The model under review builds one solid part; all positions refer to its coordinate system, in mm. Face numbers are marked on the shaded views. Give positions to 0.01 mm unless a question says otherwise; leave off trailing zeros. Order: outer loops, then holes, each group sorted by start corner. A loop starts at its lowest first (then second) coordinate and runs counter-clockwise, first axis right, second up. Notation, with made-up numbers: (6.25, 33.25) -> (42.25, 33.25) arc R25 ccw to (42.25, 53.25) -> close; hole circle Ø9 at (80, -19). An arc over 180 degrees is marked (long way). Use one line per item in the form item = value.
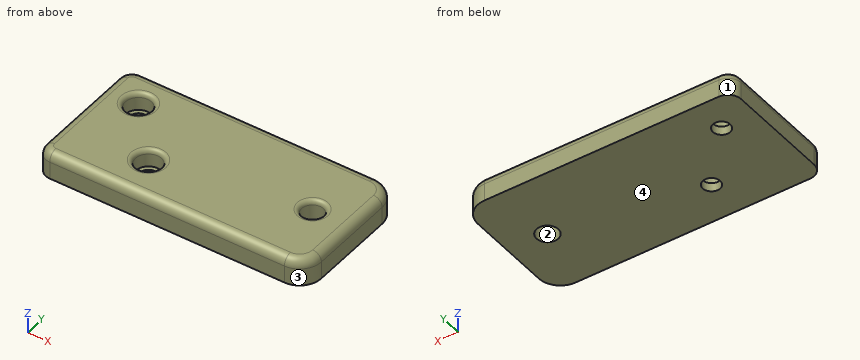
Autodesk Fusion 360 part; units mm, degrees
sketch "Sketch1" plane through (0, 0, 0) normal (0, 0, 1) x (1, 0, 0)
  circle A0 centre (0, 0) radius 2
  circle A1 centre (11.2624, -12.7341) radius 2
  circle A2 centre (11.2624, -12.7341) radius 3
  circle A3 centre (0, 0) radius 3
  line L0 (-8, 8) -> (54, 8)
  line L1 (54, 8) -> (54, -21.9327)
  line L2 (54, -21.9327) -> (-8, -21.9327)
  line L3 (-8, -21.9327) -> (-8, 8)
  circle A4 centre (45, -7) radius 2.5
  dimension "d1" = 4
  dimension "d2" = 4
  dimension "d3" = 6
  dimension "d4" = 6
  dimension "d5" = 17
  dimension "d6" = 5
extrude "Extrude1" add sketch "Sketch1" against normal blind 6 contours A2 | A3 | L0 L1 L2 L3
extrude "Extrude2" cut sketch "Sketch1" against normal blind 4 contours A2 | A3
fillet "Fillet1" radius 5 2 edges at (54, -21.9327, -3) (54, 8, -3)
fillet "Fillet2" radius 3 2 edges at (-8, -21.9327, -3) (-8, 8, -3)
fillet "Fillet3" radius 2 8 edges at (-8, -6.9663, 0) (-7.1213, 7.1213, 0) (22, 8, 0) (52.5355, 6.5355, 0) (54, -6.9663, 0) (52.5355, -20.4682, 0) (22, -21.9327, 0) (-7.1213, -21.054, 0)
fillet "Fillet4" radius 1 3 edges at (42.6692, -6.096, 0) (8.4654, -11.6493, 0) (-2.797, 1.0848, 0)
1. Add section D-D on x = 0. Give the boundary of the cut face in (y, z), then the cut area to 3 significant figures.
Values:
outline = (-21.93, -6) -> (-2, -6) -> (-2, -4) -> (-3, -4) -> (-3, -1) arc R1 ccw to (-4, 0) -> (-19.93, 0) arc R2 ccw to (-21.93, -2) -> close; (2, -6) -> (8, -6) -> (8, -2) arc R2 ccw to (6, 0) -> (4, 0) arc R1 ccw to (3, -1) -> (3, -4) -> (2, -4) -> close
area = 145 mm^2
2. For L1, parallel to Y at x = 0, z = -4.8; L2, parallel to Y at x = 46, z = -3.2; L3, parallel to X at y = -7.5, z = -5.55, list the stretches that pass through material, from the lowest coordinate up.
Values:
L1 = -21.93 to -2, 2 to 8
L2 = -21.93 to -9.29, -4.71 to 8
L3 = -8 to 42.55, 47.45 to 54
3. Add section C-C on z = -4.75. Give the boundary of the cut face in (x, y), then the cut area to 3 significant figures.
Values:
outline = (-8, -18.93) arc R3 ccw to (-5, -21.93) -> (49, -21.93) arc R5 ccw to (54, -16.93) -> (54, 3) arc R5 ccw to (49, 8) -> (-5, 8) arc R3 ccw to (-8, 5) -> close; hole circle Ø4 at (0, 0); hole circle Ø4 at (11.26, -12.73); hole circle Ø5 at (45, -7)
area = 1,800 mm^2
4. Add section A-A on x = 45. Give the boundary of the cut face in (y, z), then the cut area to 3 significant figures.
Values:
outline = (-21.93, -6) -> (-9.5, -6) -> (-9.5, -1) arc R1 ccw to (-10.5, 0) -> (-19.93, 0) arc R2 ccw to (-21.93, -2) -> close; (-4.5, -6) -> (8, -6) -> (8, -2) arc R2 ccw to (6, 0) -> (-3.5, 0) arc R1 ccw to (-4.5, -1) -> close
area = 147 mm^2
5. The part is to be moulded in two halves that separate along Y. For the marked faces 1, 2, 3 and 4, say which applies: +Y half, -Y half, draft (parallel to the pull), parting line (faces both ways), or undercut.
Values:
face_1 = +Y half
face_2 = undercut
face_3 = -Y half
face_4 = draft
6. Add section B-B on y = -7. Give the boundary of the cut face in (x, z).
Values:
outline = (-8, -6) -> (42.5, -6) -> (42.5, -1) arc R1 ccw to (41.5, 0) -> (-6, 0) arc R2 ccw to (-8, -2) -> close; (47.5, -6) -> (54, -6) -> (54, -2) arc R2 ccw to (52, 0) -> (48.5, 0) arc R1 ccw to (47.5, -1) -> close
7. For pin 1 Ø5 at (x, y) = (0, 0) entering from -Z; pin 2 Ø6.5 at (x, y) = (0, 0) entering from +Z; pin 3 Ø6.5 at (x, y) = (0.5, 0) entering from +Z, all flat-tipped, find the tip position at first contact; note any pin that passes through.
Values:
pin_1 = -6
pin_2 = -0.34
pin_3 = -0.03
